CAD build for the part. Positions are in the model's coordinates, mm. A direction names the side the tool comes from. Coordinates: 2 decimals unless noted, no trailing zeros. Order: outer loops, then holes, each group sorted by start corner. A loop starts at its lowest first (then second) coordinate and runs counter-clockwise, first axis right, second up. Notation, with made-up numbers: (54.25, 3.25) - (107.25, 3.25) arc R22 cw to (107.25, 37.25) - close; hole circle Ø2 at (89.5, 71.25). An arc over 180 degrees is marked (long way). Use one line per item in the form item = value.
```python
from build123d import *

# Parameters (mm, degrees)
F0_R        = 11.1125
F0_R_2      = 8.1915
F1_DEPTH    = 12.7
F2_R        = 11.1125
F3_DEPTH    = 19.05
F5_DEPTH    = 19.05
F6_T2_ANGLE = 169.7302536888
F6_T4_ANGLE = 84.8533787692
F6_T6_ANGLE = 84.8533787692


# Not quite as in the source:
# - a fillet or chamfer that OpenCascade refuses, or shapes differently, is made with other operations: its cross-section is extruded or revolved along the edge and cut away or added


with BuildPart() as f1:
    # F0 (on Top) → F1 (new body)
    with BuildSketch(Plane.XY):
        Circle(F0_R)
        Circle(F0_R_2, mode=Mode.SUBTRACT)
    extrude(amount=F1_DEPTH)

    # F2 (on Top) → F3 (join)
    with BuildSketch(Plane.XY):
        Circle(F2_R)
    extrude(amount=-F3_DEPTH)

    # F4 (on Front) → F5 (cut, symmetric)
    with BuildSketch(Plane.XZ):
        with BuildLine():
            Line((8.0039083969, -20.9773854417), (8.0039083969, -14.2491279898))
            ThreePointArc((8.0039083969, -14.2491279898), (6.3788176707, -7.3669087446), (0, -4.3146068702))
            ThreePointArc((0, -4.3146068702), (-6.3788176707, -7.3669087446), (-8.0039083969, -14.2491279898))
            Line((-8.0039083969, -14.2491279898), (-8.0039083969, -20.9773854417))
            Line((-8.0039083969, -20.9773854417), (8.0039083969, -20.9773854417))
        make_face()
    extrude(amount=F5_DEPTH, both=True, mode=Mode.SUBTRACT)

    # F6: fillet of radius 3.175 on 3 edges, made by hand

    # F6_s1 → F6_t2 (revolve, cut)
    with BuildSketch(Plane(origin=(0, 0, 0), x_dir=(0, 0, 1), z_dir=(0.9959867753, 0.0895005221, 0))):
        with BuildLine():
            ThreePointArc((-15.875, -11.1125), (-18.1200640303, -10.1825640303), (-19.05, -7.9375))
            Line((-19.05, -7.9375), (-19.05, -11.1125))
            Line((-19.05, -11.1125), (-15.875, -11.1125))
        make_face()
    revolve(axis=Axis((0, 0, -19.05), (0, 0, 1)), revolution_arc=F6_T2_ANGLE, mode=Mode.SUBTRACT)

    # F6_s3 → F6_t4 (revolve, cut)
    with BuildSketch(Plane(origin=(0, 0, 0), x_dir=(0, 0, 1), z_dir=(-0.9959684029, -0.08970474, 0))):
        with BuildLine():
            ThreePointArc((-15.875, -11.1125), (-18.1200640303, -10.1825640303), (-19.05, -7.9375))
            Line((-19.05, -7.9375), (-19.05, -11.1125))
            Line((-19.05, -11.1125), (-15.875, -11.1125))
        make_face()
    revolve(axis=Axis((0, 0, -19.05), (0, 0, 1)), revolution_arc=F6_T4_ANGLE, mode=Mode.SUBTRACT)

    # F6_s5 → F6_t6 (revolve, cut)
    with BuildSketch(Plane.XZ):
        with BuildLine():
            ThreePointArc((11.1125, -15.875), (10.1825640303, -18.1200640303), (7.9375, -19.05))
            Line((7.9375, -19.05), (11.1125, -19.05))
            Line((11.1125, -19.05), (11.1125, -15.875))
        make_face()
    revolve(axis=Axis((0, 0, -19.05), (0, 0, 1)), revolution_arc=F6_T6_ANGLE, mode=Mode.SUBTRACT)


solid = f1.part
```
Item 1: Drop flat-ended pins along their axis: pin 1 (5 mm diameter, centred on y = 7.5, z = 5.5, fed in from +X); pin 2 (5 mm diameter, centred on x = -2.5, y = 0.5, fed in from +Z); pin 3 (2.5 mm diameter, centred on y = -3.5, z = -17.5, fed in from +X); pin 4 (10 mm diameter, centred on x = 1.5, z = -15, fed in from -Y) (3 decimals). Give the stop position or say it passes through.
Derived:
pin_1 = 9.92
pin_2 = 0
pin_3 = 10.71
pin_4 = through
Item 2: Cut at B-B, the plane z = 1. Write the cut outline in (x, y) (1 decimal).
Derived:
outline = circle Ø22.2 at (0, 0); hole circle Ø16.4 at (0, 0)
Item 3: Cut at C-C, the plane x = 7. Write the cut outline in (y, z), plus the area to 3 significant figures.
Derived:
outline = (-8.63, -8.25) - (8.63, -8.25) - (8.63, 12.7) - (4.25, 12.7) - (4.25, 0) - (-4.25, 0) - (-4.25, 12.7) - (-8.63, 12.7) - close
area = 254 mm²
Item 4: 3-axis set-ups, long thin cutter, end or side, ignore diameter. For faces 1 (the face through (-5, -7, 12.7)), 2 (the face through (-8.004, 0, -17)): which of +Z, -Z, +X, -X, +Y, -Y reach the whole face in a straight line?
Derived:
face_1 = +Z, +X, -X, +Y, -Y
face_2 = -Z, +Y, -Y
Item 5: Drill centre lines: line 1 (Y direction, x = 0, z = 9.5); line 2 (Z direction, x = 0, y = -0.5); line 3 (Y direction, x = -5.5, z = 8.5). Where is each one in solid material? Low to high. Write a range as [from, to].
Derived:
line_1 = [-11.11, -8.19], [8.19, 11.11]
line_2 = [-4.31, 0]
line_3 = [-9.66, -6.07], [6.07, 9.66]
Item 6: Cut at A-A, the plane x = 0. Write the cut outline in (y, z), plus the area to 3 significant figures.
Derived:
outline = (-11.11, -4.31) - (11.11, -4.31) - (11.11, 12.7) - (8.19, 12.7) - (8.19, 0) - (-8.19, 0) - (-8.19, 12.7) - (-11.11, 12.7) - close
area = 170 mm²
Item 7: Two-plate mould, pull along Y, no slides. Class faces 3 (the face through (0, 0, 0)), 4 (the face through (7.8, 2.5, 6.3)), 5 (the face through (8.004, 0, -17)), 6 (the face through (-8.82, -6.76, 1.79)): +Y half, -Y half, draft (parallel to the pull), parting line (faces both ways), or undercut.
Derived:
face_3 = undercut
face_4 = undercut
face_5 = draft
face_6 = parting line
